from build123d import *

# Parameters (mm, degrees)
F1_DEPTH = 25.4


with BuildPart() as f1:
    # F0 (on Top) → F1 (new body)
    with BuildSketch(Plane.XY):
        with BuildLine():
            Line((376.802053, 154.521519), (426.124698, 182.997961))
            Line((426.124698, 182.997961), (432.474698, 186.664135))
            Line((432.474698, 186.664135), (426.124698, 197.662657))
            Line((426.124698, 197.662657), (370.452053, 165.520041))
            ThreePointArc((370.452053, 165.520041), (319.833994, 156.346437), (274.921166, 181.429912))
            Line((274.921166, 181.429912), (265.349351, 173.083034))
            ThreePointArc((265.349351, 173.083034), (317.747651, 143.81898), (376.802053, 154.521519))
        make_face()
    extrude(amount=F1_DEPTH)


solid = f1.part
The model under review builds one solid part; all positions refer to its coordinate system, in mm. A direction names the side the tool comes from. Round coordinates to 2 decimals unless told otherwise and drop trailing zeros. Loops run counter-clockwise (first coordinate to the right, second up) from the corner with the lowest first, then second, coordinate; pieces in that order, holes last. Notation, with made-up numbers: (21, 2) -> (42, 2) arc R20 cw to (42, 23) -> close; hole circle Ø11 at (85.5, 66.25). An arc over 180 degrees is marked (long way). Answer as CSV lines item,"result".
1) Add section D-D on y = 149. Write out the cut boundary in (x, z).
Geometry results:
outline,"(299.26, 0) -> (365.44, 0) -> (365.44, 25.4) -> (299.26, 25.4) -> close"
2) Add section B-B on z = 12.5. Write out the cut boundary in (x, y).
Geometry results:
outline,"(265.35, 173.08) arc R88.9 ccw to (376.8, 154.52) -> (432.47, 186.66) -> (426.12, 197.66) -> (370.45, 165.52) arc R76.2 cw to (274.92, 181.43) -> close"
3) To check wall thickness, follow line 1 along X through (y, z) = (178.5, 5); line 2 along X through (y, z) = (173, 6.5); line 3 along X through (y, z) = (154, 20.75). State the ranges of each line that lie inside material, in increasing order. Write a range as from..to.
Geometry results:
line 1,"x = 271.56..277.61, 392.93..418.33"
line 2,"x = 265.42..283.54, 383.41..408.81"
line 3,"x = 288.82..375.89"
4) Tool access review of faces 1 (the face through (399, 182, 13)), 2 (the face through (270.202, 177.315, 12.522)): name each direction out of +Z, -Z, +X, -X, +Y, -Y from which nothing blocks a thin tool from reaching the whole face with its end or side.
Geometry results:
face 1,"+Z, -Z, +Y"
face 2,"+Z, -Z, -X, +Y"
5) For P1, Ø2, axis at x = 340, z = 18.5, coming from the -Y side; P2, Ø6, axis at x = 306.5, z = 20, coming from the -Y side; P3, Ø3, axis at y = 154.5, z = 3.5, coming from the +X side, all flat-tipped, find the tip position at first contact; note any pin that passes through.
Geometry results:
P1,"stops at y = 142.86"
P2,"stops at y = 145.6"
P3,"stops at x = 379.36"
6) Add section A-A on y = 160.5. Write out the cut boundary in (x, z).
Geometry results:
outline,"(278.87, 0) -> (304.71, 0) -> (304.71, 25.4) -> (278.87, 25.4) -> close; (359.99, 0) -> (387.16, 0) -> (387.16, 25.4) -> (359.99, 25.4) -> close"
7) Add section C-C on x = 280.5. Write out the cut boundary in (y, z).
Geometry results:
outline,"(159.3, 0) -> (175.67, 0) -> (175.67, 25.4) -> (159.3, 25.4) -> close"
